from build123d import *

# Parameters (mm, degrees)
PAD010_DEPTH = 16.5
SKETCH017_R  = 0.75
PAD012_DEPTH = 1.5
SKETCH019_R  = 0.75
PAD013_DEPTH = 1.5
FILLET010_R  = 1.72


with BuildPart() as part:
    # Sketch016 → Pad010 (new body)
    with BuildSketch(Plane.XY):
        Polygon((-53.501251, -22.682802), (-50.001251, -22.682802), (-50.001251, -26.182802), (-46.501251, -26.182802), (-46.501251, -30.182802), (-50.001251, -30.182802), (-50.001251, -33.682802), (-53.501251, -33.682802), align=None)
    extrude(amount=PAD010_DEPTH)

    # Sketch017 (on Face10 of Pad010) → Pad012 (join)
    with BuildSketch(Plane.XY.offset(16.5)):
        with Locations((-51.751251, -24.932802)):
            Circle(SKETCH017_R)
        with Locations((-51.751251, -31.432802)):
            Circle(SKETCH017_R)
        with Locations((-48.501251, -28.182802)):
            Circle(SKETCH017_R)
    extrude(amount=PAD012_DEPTH)

    # Sketch019 → Pad013 (join)
    with BuildSketch(Plane(origin=(0, 0, 0), x_dir=(1, 0, 0), z_dir=(0, 0, -1))):
        with Locations((-51.751251, 31.432802)):
            Circle(SKETCH019_R)
        with Locations((-51.751251, 24.932802)):
            Circle(SKETCH019_R)
        with Locations((-48.236244, 28.182802)):
            Circle(SKETCH019_R)
    extrude(amount=PAD013_DEPTH)

    # Fillet010
    fillet010_edges = [part.edges().sort_by_distance(p)[0] for p in [
        (-50.001251, -30.182802, 8.25),
        (-50.001251, -33.682802, 8.25),
        (-46.501251, -30.182802, 8.25),
        (-46.501251, -26.182802, 8.25),
        (-50.001251, -22.682802, 8.25),
        (-50.001251, -26.182802, 8.25),
    ]]
    fillet(fillet010_edges, radius=FILLET010_R)


with BuildPart() as part_1:
    # Body003 placement: moved
    add(part.part.moved(Location((-1.4, 15.2, 11.1))))


solid = part_1.part
Geometry check sheet. Reference: the model listing, model coordinates, mm. A direction names the side the tool comes from. Round coordinates to 2 decimals unless told otherwise and drop trailing zeros. Loops run counter-clockwise (first coordinate to the right, second up) from the corner with the lowest first, then second, coordinate; pieces in that order, holes last.
Item 1: Cross-section at A-A on z = 24.5. Record the boundary of the cut face in (x, y).
Item 2: Thickness scan on line 1 (Z direction, x = -51.25, y = -12); line 2 (X direction, y = -16, z = 22.5); line 3 (X direction, y = -15.25, z = 15.25). Record the ranges inside material, lowest first.
Item 3: Cross-section at C-C on y = -16. Record the boundary of the cut face in (x, z).
Item 4: Cross-section at D-D on y = -14.5. Record the boundary of the cut face in (x, z), then the cut area to 3 significant figures.
Item 5: Access from +Z, -Z, +X, -X, +Y, -Y to the whole of each face (thin tool, end or side, straight path). Record for faces 1 (the cylindrical face through (-50.91, -15.5, 19.47)), 2 (the cylindrical face through (-52.436, -9.508, 28.34)), 3 (the cylindrical face through (-52.436, -9.958, 10.36)).
Item 6: Cross-section at B-B on y = -10.25. Record the boundary of the cut face in (x, z), then the cut area to 3 significant figures.
Item 7: Mould release check, pull along Y, two halves, no side actions. Record for faces 4 (the cylindrical face through (-52.46, -16.52, 28.34)), 5 (the flat face through (-53, -16, 29.1)), 6 (the cylindrical face through (-48.392, -14.466, 19.466)): pulls with the +Y half, pulls with the -Y half, needs draft (parallel to the pull), parting line crosses it, or undercut.
Answer sheet:
1. outline: (-54.9, -18.48) - (-53.12, -18.48) arc R1.72 ccw to (-51.4, -16.76) - (-51.4, -16.7) arc R1.72 cw to (-49.68, -14.98) - (-49.62, -14.98) arc R1.72 ccw to (-47.9, -13.26) - (-47.9, -12.7) arc R1.72 ccw to (-49.62, -10.98) - (-49.68, -10.98) arc R1.72 cw to (-51.4, -9.26) - (-51.4, -9.2) arc R1.72 ccw to (-53.12, -7.48) - (-54.9, -7.48) - close
2. line 1: z = 11.1 to 27.6
2. line 2: x = -54.9 to -51.25
2. line 3: x = -54.9 to -50.6
3. outline: (-54.9, 11.1) - (-53.86, 11.1) - (-53.86, 9.6) - (-52.44, 9.6) - (-52.44, 11.1) - (-51.25, 11.1) - (-51.25, 27.6) - (-52.44, 27.6) - (-52.44, 29.1) - (-53.86, 29.1) - (-53.86, 27.6) - (-54.9, 27.6) - close
4. outline: (-54.9, 11.1) - (-48.43, 11.1) - (-48.43, 27.6) - (-54.9, 27.6) - close
4. area: 107 mm2
5. face 1: +Z, -Z, +X, -Y
5. face 2: +Z
5. face 3: -Z
6. outline: (-54.9, 11.1) - (-53.69, 11.1) - (-53.69, 9.6) - (-52.61, 9.6) - (-52.61, 11.1) - (-51.09, 11.1) - (-51.09, 27.6) - (-52.61, 27.6) - (-52.61, 29.1) - (-53.69, 29.1) - (-53.69, 27.6) - (-54.9, 27.6) - close
6. area: 66.1 mm2
7. face 4: undercut
7. face 5: needs draft
7. face 6: pulls with the -Y half
